Geometry: see drawing. Coordinates: mm, zero at the bounding-box minimum. A direction names the side the tool comes from. Round coordinates to 2 decimals unless told otherwise and drop trailing zeros. Loops run counter-clockwise (first coordinate to the right, second up) from the corner with the lowest first, then second, coordinate; pieces in that order, holes last.
(1) Section B-B, the plane y = 13. Count the separate pieces of the cut face and the enclosed holes in it, plus the area to 3 significant figures.
(2) First-contact query: pin 1 Ø5 at (y, z) = (19, 29.5) entering from -X; pin 2 Ø1 at (y, z) = (31, 62.5) entering from -X; pin 3 Ø1.5 at (y, z) = (8, 61) entering from +X. Flat tips, straight axial feed; report the tip coordinate or a pass-through.
(3) Section D-D, the plane z = 65. Return the cut outline in (x, y).
(4) Material intervals for probe 1 along X at (y, z) = (26, 12); probe 2 along X at (y, z) = (29, 67.5); probe 3 along Z at (x, y) = (91.5, 12) (1 decimal), sorted ascending.
(5) Mould query, pull axis X, two halves, no side actions, for the marked faces 1, 2, 3 and 4. Classes: pulls with the +X half, pulls with the -X half, needs draft (parallel to the pull), parting line crosses it, or undercut.
(6) Set-up query: the marked faces 5 and 6. Return all of +Z, -Z, +X, -X, +Y, -Y with unobstructed straight access to the full face (end or side cutting, diameter ignored); none if empty.
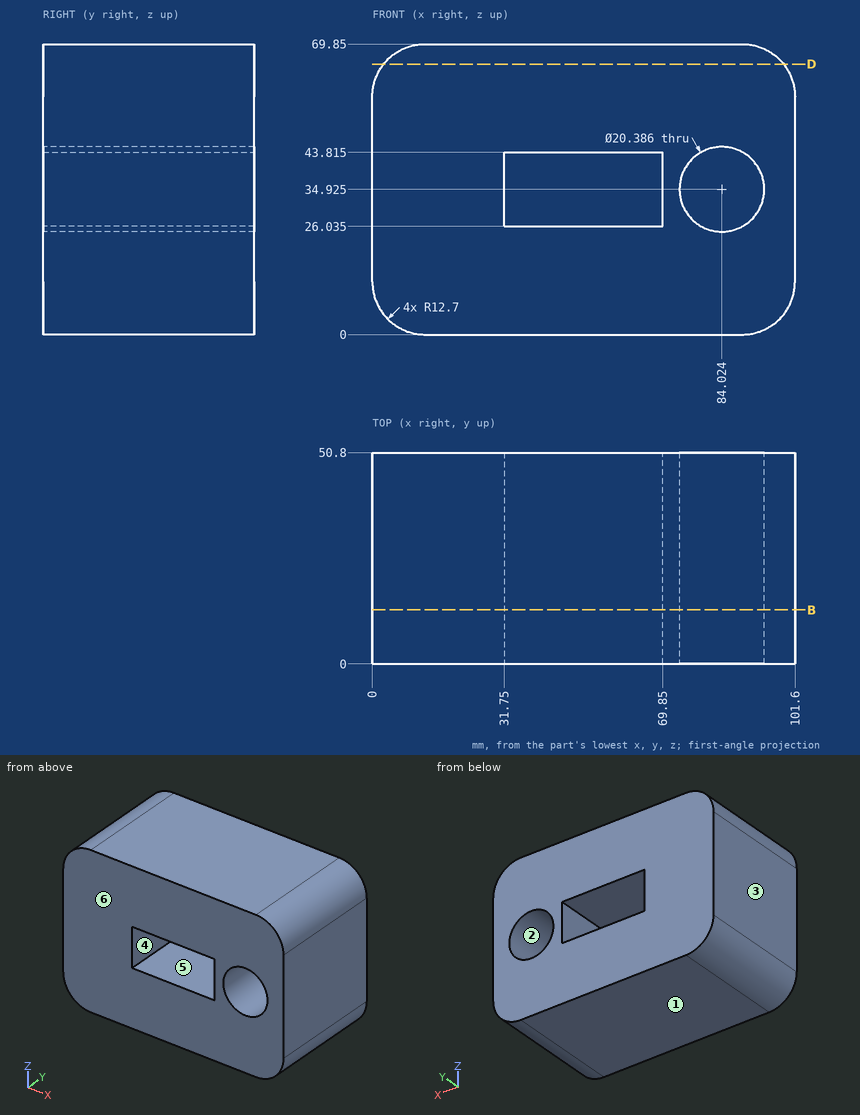
Output values:
1. separate pieces: 1
1. enclosed holes: 2
1. area: 5,950 mm2
2. pin 1: stops at x = 0
2. pin 2: stops at x = 0.96
2. pin 3: stops at x = 101.22
3. outline: (2.72, 0) - (98.88, 0) - (98.88, 50.8) - (2.72, 50.8) - close
4. probe 1: x = 0.02 to 101.58
4. probe 2: x = 5.34 to 96.26
4. probe 3: z = 0.3 to 28, 41.9 to 69.6
5. face 1: needs draft
5. face 2: undercut
5. face 3: pulls with the -X half
5. face 4: undercut
6. face 5: +Y, -Y
6. face 6: +Z, -Z, +X, -X, -Y
